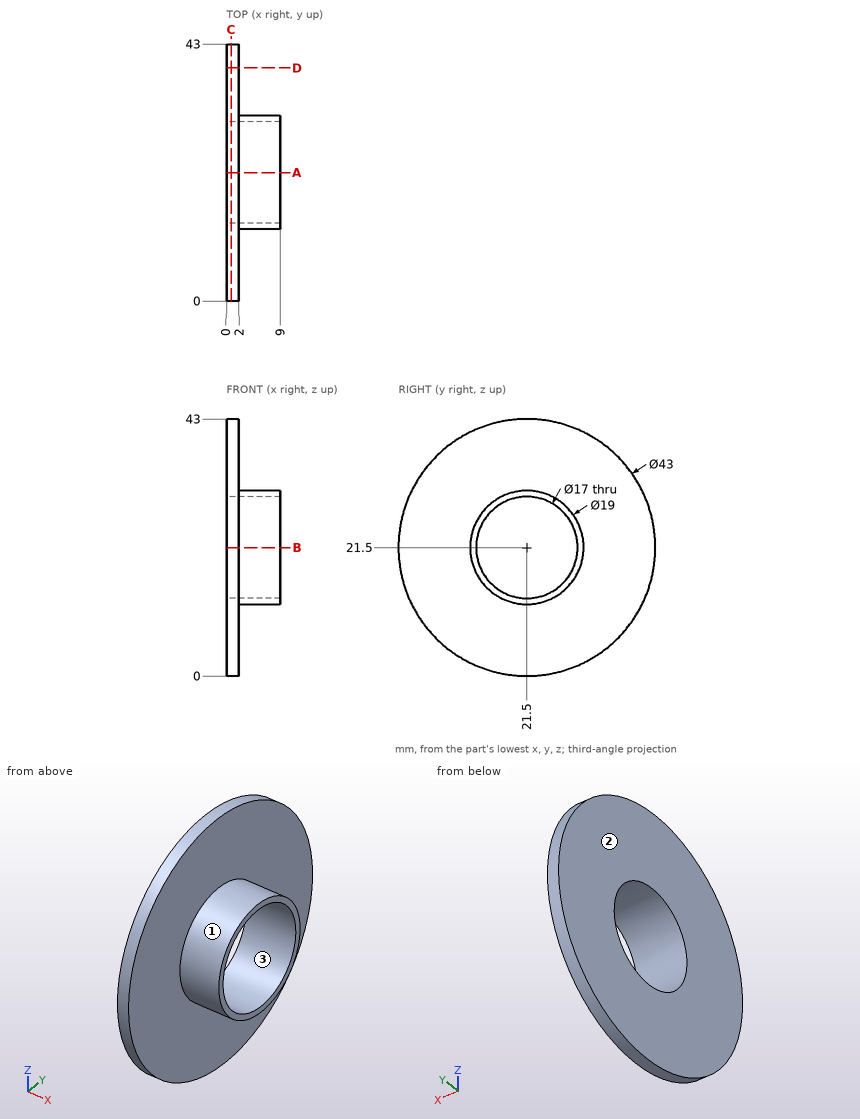
Here's the drawing with two shaded views (mm, measured from the low corner). I have some questions. Give positions to 0.01 mm unless a question says otherwise; leave off trailing zeros. Order: outer loops, then holes, each group sorted by start corner. A loop starts at its lowest first (then second) coordinate and runs counter-clockwise, first axis right, second up. Notation, with made-up numbers: (-27, 49.25) -> (23, 49.25) arc R28 cw to (23, 74.25) -> close; hole circle Ø5 at (-32, 65.5). An arc over 180 degrees is marked (long way). One line per item, written item: value. Start each with the question number.
1. Imagine slicing it at C-C, the plane x = 0.75. List the corners of the cut face in (y, z) for me.
2. Imagine slicing it at D-D, the plane y = 39. List the corners of the cut face in (x, z) for me, plus the area to 3 significant figures.
3. Imagine slicing it at A-A, the plane y = 21.5. List the corners of the cut face in (x, z) for me.
4. Will these pins go through, and if not, where does the flat tip stop? pin 1 Ø5 at (x, y) = (1, 15) entering from -Z; pin 2 Ø1.5 at (y, z) = (29.5, 29) entering from +X; pin 3 Ø5 at (x, y) = (7.5, 18) entering from -Z.
5. We'd pull the mould along Y, two halves only. Please class the marked faces 1, 2 and 3: released by +Y, released by -Y, zero draft, split by the parting line, or undercut.
6. I need wall thicknesses on probe 1 along Y at (x, z) = (6.75, 21.5); probe 2 along Y at (x, z) = (3, 27); probe 3 along X at (y, z) = (27.5, 13.5). Which ranges of each line are inside material? Lowest first, please. Write a range as from..to.
Values follow:
1. outline: circle Ø43 at (21.5, 21.5); hole circle Ø17 at (21.5, 21.5)
2. outline: (0, 9.01) -> (2, 9.01) -> (2, 33.99) -> (0, 33.99) -> close
2. area: 50.0 mm2
3. outline: (0, 0) -> (2, 0) -> (2, 12) -> (9, 12) -> (9, 13) -> (0, 13) -> close; (0, 30) -> (9, 30) -> (9, 31) -> (2, 31) -> (2, 43) -> (0, 43) -> close
4. pin 1: stops at z = 0.38
4. pin 2: stops at x = 2
4. pin 3: stops at z = 12.05
5. face 1: split by the parting line
5. face 2: zero draft
5. face 3: undercut
6. probe 1: y = 12..13, 30..31
6. probe 2: y = 13.75..15.02, 27.98..29.25
6. probe 3: x = 0..2
